Could you check a few things on this drawing? It's one solid part, dimensions in mm from its lowest x, y, z. Round coordinates to 2 decimals unless told otherwise and drop trailing zeros. Order: outer loops, then holes, each group sorted by start corner. A loop starts at its lowest first (then second) coordinate and runs counter-clockwise, first axis right, second up. Notation, with made-up numbers: (-31.5, -3) - (4.5, -3) arc R20 cw to (4.5, 6) - close; hole circle Ø10 at (5.5, 88.5). An arc over 180 degrees is marked (long way). Use one line per item in the form item = value.
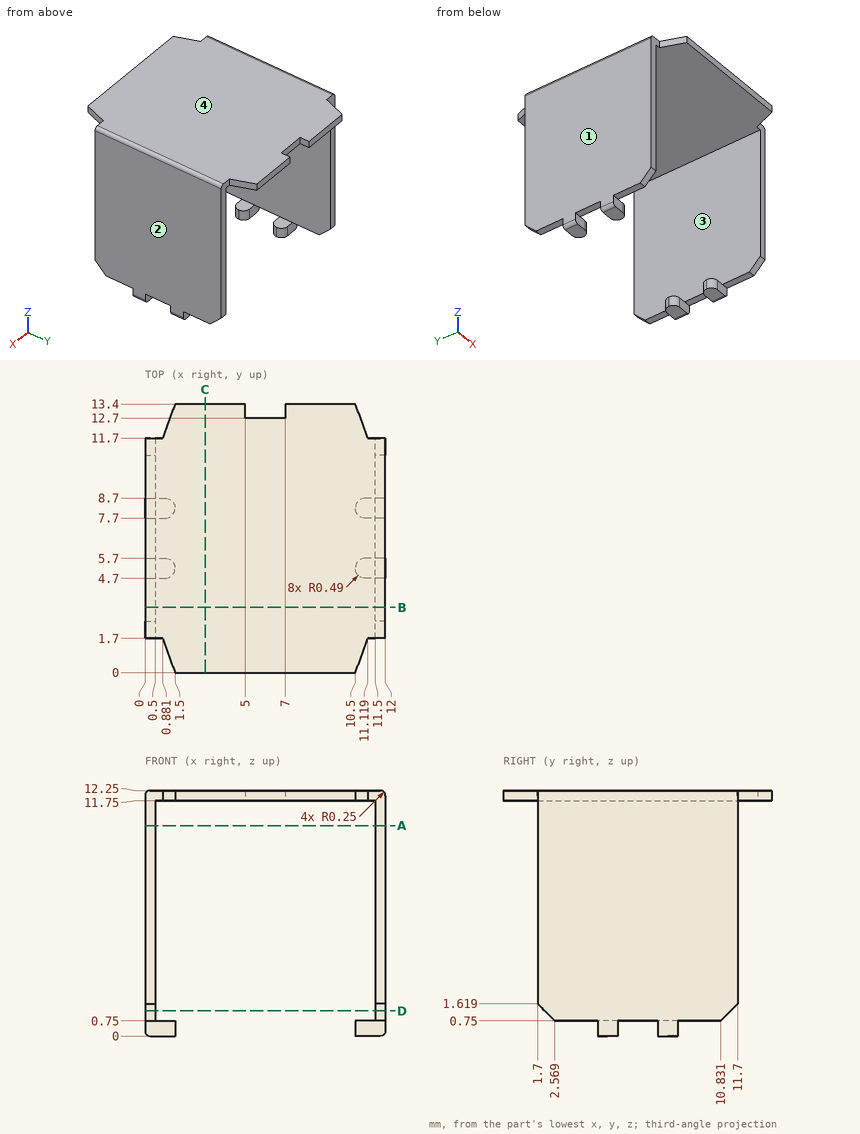
Item 1: If we mould it in two halves opening along X, with no side actions, what happens to the marked faces 1, 2, 3 and 4? For each: released by +X, released by -X, zero draft, split by the parting line, or undercut.
Found:
face_1 = released by -X
face_2 = released by +X
face_3 = undercut
face_4 = zero draft
Item 2: Imagine slicing it at B-B on y = 3.25. Please give me the cut outline in (x, z).
Found:
outline = (0, 0.75) - (0.5, 0.75) - (0.5, 11.75) - (11.5, 11.75) - (11.5, 0.75) - (12, 0.75) - (12, 12) arc R0.25 ccw to (11.75, 12.25) - (0.25, 12.25) arc R0.25 ccw to (0, 12) - close
Item 3: Imagine slicing it at C-C on x = 3. Please give me the cut outline in (y, z).
Found:
outline = (0, 11.75) - (13.4, 11.75) - (13.4, 12.25) - (0, 12.25) - close
Item 4: Imagine slicing it at A-A on z = 10.5. Please give me the cut outline in (x, y), plus the area to 3 significant figures.
Found:
outline = (0, 1.7) - (0.5, 1.7) - (0.5, 11.7) - (0, 11.7) - close; (11.5, 1.7) - (12, 1.7) - (12, 11.7) - (11.5, 11.7) - close
area = 10.0 mm2
Item 5: Will these pins go through, and if not, where does the flat tip stop? P1, Ø0.6, axis at x = 0.5, z = 0.5, coming from the +Y side; P2, Ø0.7, axis at x = 11.5, z = 4.5, coming from the -Y side; P3, Ø3, axis at x = 8.5, z = 1.5, coming from the -Y side; P4, Ø3.5, axis at x = 3.5, y = 5.5, coming from the -Z side.
Found:
P1 = 10.88
P2 = 1.7
P3 = through
P4 = 11.75
Item 6: Imagine slicing it at D-D on z = 1.25. Please give me the cut outline in (x, y).
Found:
outline = (0, 2.07) - (0.5, 2.07) - (0.5, 11.33) - (0, 11.33) - close; (11.5, 2.07) - (12, 2.07) - (12, 11.33) - (11.5, 11.33) - close
Item 7: I need wall thicknesses on L1, parallel to X at y = 9.25, z = 1.75; L2, parallel to Z at x = 1.5, y = 11.5; L3, parallel to Z at x = 11.75, y = 7.5. Which ranges of each line are inside material? Lowest first, please.
Found:
L1 = 0 to 0.5, 11.5 to 12
L2 = 11.75 to 12.25
L3 = 0.75 to 12.25
